Source: CAD feature listing. Evaluate the final solid. Frame: model axes, mm. Coordinates: 2 decimals unless noted, no trailing zeros. Order: outer loops, then holes, each group sorted by start corner. A loop starts at its lowest first (then second) coordinate and runs counter-clockwise, first axis right, second up.
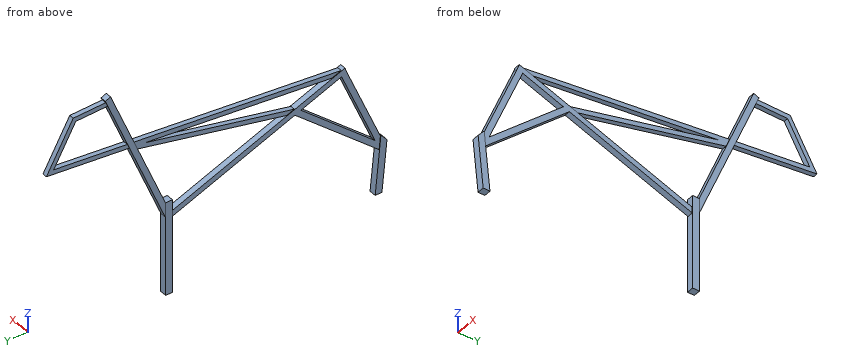
```python
from build123d import *

# Parameters (mm, degrees)
F2_DEPTH = 6
F3_DEPTH = 5
F4_DEPTH = 4


with BuildPart() as f2:
    # F1 (on Right) → F2 (new body, symmetric)
    with BuildSketch(Plane.YZ):
        Polygon((6, 168.0537815686), (-6, 168.0537815686), (-6, 147.4344787753), (-6, 136.8235857408), (-6, 0), (6, 0), (6, 141.4846799699), align=None)
    extrude(amount=F2_DEPTH, both=True)



with BuildPart() as f2b:
    # F1 (on Right) → F2, piece 2 (new body, symmetric)
    with BuildSketch(Plane.YZ):
        Polygon((-366.1312568474, 0), (-373.8555777285, 78.8196008275), (-375.0700772329, 91.2124529134), (-376.1697828669, 102.433938974), (-376.3721973614, 104.499393), (-387.1445919312, 91.3862120271), (-378.1887431526, 0), align=None)
    extrude(amount=F2_DEPTH, both=True)


with BuildPart() as f2_1:
    add(f2.part)

    add(f2b.part)  # F3 merges F2b
    # F1 (on Right) → F3 (join, symmetric)
    with BuildSketch(Plane.YZ):
        Polygon((54.9115302543, 288.4513945022), (6, 168.0537815686), (6, 141.4846799699), (69.1811610546, 297.0075379505), (72.6501883928, 305.5466821674), (107.7718487622, 392), (111.0218487622, 400), (112.5273569501, 403.7058663085), (103.2626911788, 407.469636778), (61.2320620859, 304.0096267031), (57.7630347477, 295.4704824861), align=None)
        Polygon((-6, 136.8235857408), (-6, 147.4344787753), (-210.4892851655, 219.9951928663), (-223.9719705091, 224.7793715366), (-290.9143972643, 248.5331358691), (-307.4065665233, 254.3851959287), (-313.2799449629, 256.4692979557), (-316.6240434146, 247.0450205009), (-307.1881482882, 243.6967996495), (-235.0141298479, 218.086664074), (-224.3114881972, 214.2889525205), align=None)
        Polygon((-373.8555777285, 78.8196008275), (-224.3114881972, 214.2889525205), (-235.0141298479, 218.086664074), (-366.9451312979, 98.5726980545), (-375.0700772329, 91.2124529134), align=None)
        Polygon((-366.9451312979, 98.5726980545), (-307.1881482882, 243.6967996495), (-316.6240434146, 247.0450205009), (-376.1697828669, 102.433938974), (-375.0700772329, 91.2124529134), align=None)
    extrude(amount=F3_DEPTH, both=True)

    # F1 (on Right) → F4 (join, symmetric)
    with BuildSketch(Plane.YZ):
        Polygon((41.7213857169, 293.3110297319), (57.7630347477, 295.4704824861), (61.2320620859, 304.0096267031), (-307.4065665233, 254.3851959287), (-290.9143972643, 248.5331358691), align=None)
        Polygon((-210.4892851655, 219.9951928663), (54.9115302543, 288.4513945022), (57.7630347477, 295.4704824861), (41.7213857169, 293.3110297319), (-223.9719705091, 224.7793715366), align=None)
        Polygon((72.6501883928, 305.5466821674), (69.1811610546, 297.0075379505), (216.4195260905, 316.8280870899), (203.5804739095, 323.1719129101), align=None)
        Polygon((203.5804739095, 323.1719129101), (216.4195260905, 316.8280870899), (168.8927187133, 400), (164.2501384295, 392), align=None)
        Polygon((164.2501384295, 392), (168.8927187133, 400), (111.0218487622, 400), (107.7718487622, 392), align=None)
    extrude(amount=F4_DEPTH, both=True)


solid = f2_1.part
```
Q1. Material intervals for line 1 along Z through (x, y) = (2, -149); line 2 along Z through (x, y) = (2.5, -76); line 3 along X through (y, z) = (-341, 176.5), sorted ascending.
Solutions:
line 1: z = 187.57 to 198.18, 235.86 to 244.12, 267.64 to 275.71
line 2: z = 161.66 to 172.27, 254.68 to 262.95, 277.46 to 285.54
line 3: x = -5 to 5
Q2. Section query D-D on z = 128. Output: boundary loops of the cut face in (x, y).
Solutions:
outline: (-6, -6) - (6, -6) - (6, 6) - (-6, 6) - close; (-5, -365.64) - (5, -365.64) - (5, -354.83) - (-5, -354.83) - close; (-5, -334.46) - (5, -334.46) - (5, -319.57) - (-5, -319.57) - close
Q3. Section query C-C on y = -142. Output: boundary loops of the cut face in (x, z).
Solutions:
outline: (-5, 185.08) - (5, 185.08) - (5, 195.69) - (-5, 195.69) - close; (-4, 237.66) - (4, 237.66) - (4, 245.92) - (-4, 245.92) - close; (-4, 268.58) - (4, 268.58) - (4, 276.65) - (-4, 276.65) - close
Q4. Pin query (flat end, axial travel): P1, Ø2.5, axis at x = -1, y = 133.5, coming from the +Z side; P2, Ø3, axis at x = 0, y = -210, coming from the +Z side; P3, Ø6, axis at x = 2, y = -2.5, coming from the +Z side. Return the tip coordinate at first contact, or that it passes through.
Solutions:
P1: stops at z = 400
P2: stops at z = 267.7
P3: stops at z = 295.83
Q5. Section query B-B on y = 48. Output: boundary loops of the cut face in (x, z).
Solutions:
outline: (-5, 244.87) - (5, 244.87) - (5, 271.44) - (-5, 271.44) - close; (-4, 286.67) - (4, 286.67) - (4, 302.23) - (-4, 302.23) - close
Q6. Section query A-A on z = 54.5. Output: boundary loops of the cut face in (x, y).
Solutions:
outline: (-6, -383.53) - (6, -383.53) - (6, -371.47) - (-6, -371.47) - close; (-6, -6) - (6, -6) - (6, 6) - (-6, 6) - close
